from build123d import *

# Parameters (mm, degrees)
BOSS_EXTRUDE1_DEPTH = 5
SKETCH2_R           = 1
CUT_EXTRUDE1_DEPTH  = 5


with BuildPart() as part:
    # Sketch1 → Boss-Extrude1 (new body)
    with BuildSketch(Plane.XY):
        with BuildLine():
            Line((-7, 0), (-5, 0))
            ThreePointArc((-5, 0), (0, 5), (5, 0))
            Line((5, 0), (7, 0))
            Line((7, 0), (12, 0))
            Line((12, 0), (12, 3))
            Line((12, 3), (6.32455532, 3))
            ThreePointArc((6.32455532, 3), (0, 7), (-6.32455532, 3))
            Line((-6.32455532, 3), (-12, 3))
            Line((-12, 3), (-12, 0))
            Line((-12, 0), (-7, 0))
        make_face()
    extrude(amount=BOSS_EXTRUDE1_DEPTH)

    # Sketch2 → Cut-Extrude1 (cut)
    with BuildSketch(Plane(origin=(0, 3, 0), x_dir=(1, 0, 0), z_dir=(0, 1, 0))):
        with Locations(Location((-9.5, -2.5, 0), (0, 0, 270))):
            Circle(SKETCH2_R)
        with Locations(Location((9.5, -2.5, 0), (0, 0, 180))):
            Circle(SKETCH2_R)
    extrude(amount=-CUT_EXTRUDE1_DEPTH, mode=Mode.SUBTRACT)


solid = part.part
Here's how the part is built. I have some questions about the finished solid (model axes, mm). A direction names the side the tool comes from. Round coordinates to 2 decimals unless told otherwise and drop trailing zeros. Write each loop counter-clockwise with the first axis right and the second up, starting at its lowest first coordinate (ties: lowest second). Pieces come first, ordered by that corner, then holes.
1. Suppose I cut it at D-D (z = 0.45). List the corners of the cut face in (x, y) for me, and give its area (3 significant figures).
2. I need wall thicknesses on L1, parallel to Z at x = 9.5, y = 0.85; L2, parallel to X at y = 1.5, z = 2.8; L3, parallel to Y at x = 10, z = 3.7. Which ranges of each line are inside material? Lowest first, please.
3. Suppose I cut it at C-C (z = 2.5). List the corners of the cut face in (x, y) for me, and give its area (3 significant figures).
4. Suppose I cut it at B-B (y = 1.75). List the corners of the cut face in (x, z) for me.
5. Suppose I cut it at A-A (x = -9.5). List the corners of the cut face in (y, z) for me, and give its area (3 significant figures).
6. Will these pins go through, and if not, where does the flat tip stop? pin 1 Ø1 at (x, z) = (0, 3.5) entering from -Y; pin 2 Ø2.5 at (x, z) = (-9.5, 2.5) entering from +Y.
7. If we mould it in two halves opening along X, with no side actions, what happens to faces 1 (the flat face through (-8, 3, 2)), 2 (the cylindrical face through (-8.51, 1.52, 2.37)), 3 (the flat face through (12, 1, 2))? For each: released by +X, released by -X, zero draft, split by the parting line, or undercut.
8. For faces 4 (the flat face through (9, 3, 1)), 5 (the flat face through (-8.5, 0, 1.9)), which set-ups out of +Z, -Z, +X, -X, +Y, -Y let a thin tool reach every point of the face, with its end or its side?
Answer sheet:
1. outline: (-12, 0) - (-5, 0) arc R5 cw to (5, 0) - (12, 0) - (12, 3) - (6.32, 3) arc R7 ccw to (-6.32, 3) - (-12, 3) - close
1. area: 69.0 mm2
2. L1: z = 0 to 1.5, 3.5 to 5
2. L2: x = -12 to -10.45, -8.55 to -4.77, 4.77 to 8.55, 10.45 to 12
2. L3: y = 0 to 3
3. outline: (-12, 0) - (-10.5, 0) - (-10.5, 3) - (-12, 3) - close; (-8.5, 0) - (-5, 0) arc R5 cw to (5, 0) - (8.5, 0) - (8.5, 3) - (6.32, 3) arc R7 ccw to (-6.32, 3) - (-8.5, 3) - close; (10.5, 0) - (12, 0) - (12, 3) - (10.5, 3) - close
3. area: 57.0 mm2
4. outline: (-12, 0) - (-4.68, 0) - (-4.68, 5) - (-12, 5) - close; (4.68, 0) - (12, 0) - (12, 5) - (4.68, 5) - close; hole circle Ø2 at (-9.5, 2.5); hole circle Ø2 at (9.5, 2.5)
5. outline: (0, 0) - (3, 0) - (3, 1.5) - (0, 1.5) - close; (0, 3.5) - (3, 3.5) - (3, 5) - (0, 5) - close
5. area: 9.00 mm2
6. pin 1: stops at y = 4.97
6. pin 2: stops at y = 3
7. face 1: zero draft
7. face 2: undercut
7. face 3: released by +X
8. face 4: +Z, -Z, +X, +Y
8. face 5: +Z, -Z, +X, -X, -Y
